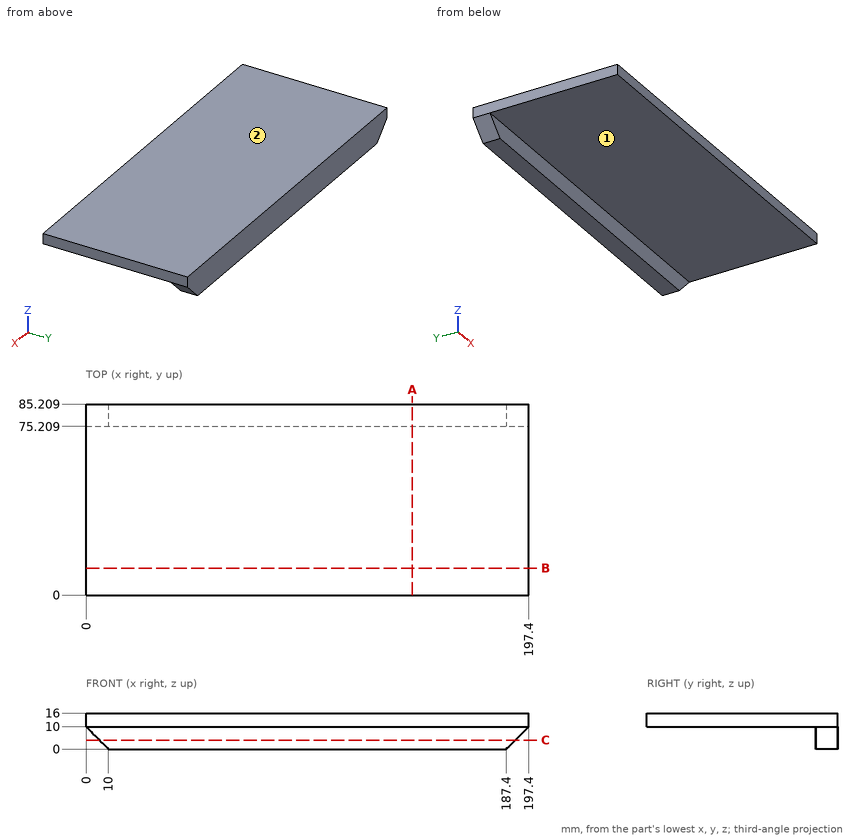
The figure shows three views and two pictorial views of one solid part (mm, origin at its lowest corner). Answer the questions. A direction names the side the tool comes from. Coordinates: 2 decimals unless noted, no trailing zeros. Write each loop counter-clockwise with the first axis right and the second up, starting at its lowest first coordinate (ties: lowest second). Pieces come first, ordered by that corner, then holes. Notation, with made-up numbers: (31.5, 4.25) -> (60.5, 4.25) arc R20 ccw to (60.5, 16.25) -> close; hole circle Ø9 at (-16, 68). An arc over 180 degrees is marked (long way). Answer as a JSON object with one key per item and string values.
Q1. A flat-ended cylindrical pin translates along its axis: pin 1 Ø1 at (x, y) = (71, 18.5) entering from -Z. Find the tip coordinate at first contact, or state that the pin passes through.
The answers:
{"pin 1": "stops at z = 10"}
Q2. The part is cut by section A-A on x = 145.5. Give the vertices of the cut face in (y, z), then the cut area to 3 significant figures.
The answers:
{"outline": "(0, 10) -> (75.21, 10) -> (75.21, 0) -> (85.21, 0) -> (85.21, 16) -> (0, 16) -> close", "area": "611 mm2"}
Q3. The part is cut by section C-C on z = 4. Give the vertices of the cut face in (x, y).
The answers:
{"outline": "(6, 75.21) -> (191.4, 75.21) -> (191.4, 85.21) -> (6, 85.21) -> close"}
Q4. The part is cut by section B-B on y = 12. Give the vertices of the cut face in (x, z), then the cut area to 3 significant figures.
The answers:
{"outline": "(0, 10) -> (197.4, 10) -> (197.4, 16) -> (0, 16) -> close", "area": "1,180 mm2"}
Q5. A tool of negligible diameter and unlimited length cuts with its end or side. For the marked faces 1 and 2, from which of +Z, -Z, +X, -X, +Y, -Y can it reach the whole face along a straight path? Write none if from no direction.
The answers:
{"face 1": "-Z, +X, -X, -Y", "face 2": "+Z, +X, -X, +Y, -Y"}
Q6. Consider line 1 (Z direction, x = 178.5, y = 14.5); line 2 (Y direction, x = 97, z = 9); line 3 (X direction, y = 81.5, z = 8). Determine where each line is inside the solid, lowest interval first. Write a range as [from, to].
The answers:
{"line 1": "z = [10, 16]", "line 2": "y = [75.21, 85.21]", "line 3": "x = [2, 195.4]"}
